```python
from build123d import *

# Parameters (mm, degrees)
BOSS_EXTRUDE1_DEPTH = 12
SKETCH3_R           = 1.184698277
CUT_EXTRUDE3_DEPTH  = 5
BOSS_EXTRUDE6_DEPTH = 12
CUT_EXTRUDE4_DEPTH  = 12
SKETCH10_R          = 1.184698277
CUT_EXTRUDE5_DEPTH  = 12
CUT_EXTRUDE7_DEPTH  = 19


with BuildPart() as part:
    # Sketch1 → Boss-Extrude1 (new body)
    with BuildSketch(Plane.XY):
        with BuildLine():
            Line((-4.775747962, -5), (-3.406624892, -5))
            ThreePointArc((-3.406624892, -5), (-6.090000101, 0), (-3.406624892, 5))
            Line((-3.406624892, 5), (3.226624689, 5))
            ThreePointArc((3.226624689, 5), (5.909999899, 0), (3.226624689, -5))
            Line((3.226624689, -5), (4.595747759, -5))
            ThreePointArc((4.595747759, -5), (-0.090000101, 6.852461821), (-4.775747962, -5))
        make_face()
        with BuildLine():
            Line((11.597073435, -5), (4.595747759, -5))
            ThreePointArc((4.595747759, -5), (3.939029098, -5.542847348), (3.220019991, -6))
            Line((3.220019991, -6), (11.597073435, -6))
            Line((11.597073435, -6), (11.597073435, -5))
        make_face()
        with BuildLine():
            Line((3.226624689, -5), (-3.406624892, -5))
            Line((-3.406624892, -5), (-4.775747962, -5))
            ThreePointArc((-4.775747962, -5), (-4.119029301, -5.542847348), (-3.400020194, -6))
            Line((-3.400020194, -6), (3.220019991, -6))
            ThreePointArc((3.220019991, -6), (3.939029098, -5.542847348), (4.595747759, -5))
            Line((4.595747759, -5), (3.226624689, -5))
        make_face()
        with BuildLine():
            ThreePointArc((-3.400020194, -6), (-4.119029301, -5.542847348), (-4.775747962, -5))
            Line((-4.775747962, -5), (-11.777073637, -5))
            Line((-11.777073637, -5), (-11.777073637, -6))
            Line((-11.777073637, -6), (-3.400020194, -6))
        make_face()
    extrude(amount=BOSS_EXTRUDE1_DEPTH)

    # Sketch3 → Cut-Extrude3 (cut)
    with BuildSketch(Plane(origin=(0, -5, 0), x_dir=(1, 0, 0), z_dir=(0, 1, 0))):
        with Locations((-9.627163284, -9.379788166)):
            Circle(SKETCH3_R)
        with Locations((9.447163082, -9.379788166)):
            Circle(SKETCH3_R)
        with Locations((9.447163082, -2.620211834)):
            Circle(SKETCH3_R)
        with Locations((-9.627163284, -2.620211834)):
            Circle(SKETCH3_R)
    extrude(amount=-CUT_EXTRUDE3_DEPTH, mode=Mode.SUBTRACT)

    # Sketch7 → Boss-Extrude6 (add)
    with BuildSketch(Plane.XY.offset(12)):
        with BuildLine():
            ThreePointArc((5.456145908, -5), (0, 7.400643767), (-5.456145908, -5))
            Line((-5.456145908, -5), (-4.775747962, -5))
            ThreePointArc((-4.775747962, -5), (-0.090000101, 6.852461821), (4.595747759, -5))
            Line((4.595747759, -5), (5.456145908, -5))
        make_face()
        with BuildLine():
            Line((-4.33238135, -6), (-11.777073637, -6))
            Line((-11.777073637, -6), (-11.777073637, -6.756480667))
            Line((-11.777073637, -6.756480667), (-3.019850519, -6.756480667))
            ThreePointArc((-3.019850519, -6.756480667), (-3.695523524, -6.411913447), (-4.33238135, -6))
        make_face()
        with BuildLine():
            Line((4.33238135, -6), (-4.33238135, -6))
            ThreePointArc((-4.33238135, -6), (-3.695523524, -6.411913447), (-3.019850519, -6.756480667))
            Line((-3.019850519, -6.756480667), (3.019850519, -6.756480667))
            ThreePointArc((3.019850519, -6.756480667), (3.695523524, -6.411913447), (4.33238135, -6))
        make_face()
        with BuildLine():
            Line((11.597073435, -6), (4.33238135, -6))
            ThreePointArc((4.33238135, -6), (3.695523524, -6.411913447), (3.019850519, -6.756480667))
            Line((3.019850519, -6.756480667), (11.597073435, -6.756480667))
            Line((11.597073435, -6.756480667), (11.597073435, -6))
        make_face()
    extrude(amount=-BOSS_EXTRUDE6_DEPTH)

    # Sketch9 → Cut-Extrude4 (cut)
    with BuildSketch(Plane.XY.offset(12)):
        with BuildLine():
            Line((-3.476794678, 5), (3.476794678, 5))
            ThreePointArc((3.476794678, 5), (6.090000101, 0), (3.476794678, -5))
            Line((3.476794678, -5), (-3.476794678, -5))
            ThreePointArc((-3.476794678, -5), (-6.090000101, 0), (-3.476794678, 5))
        make_face()
    extrude(amount=-CUT_EXTRUDE4_DEPTH, mode=Mode.SUBTRACT)

    # Sketch10 → Cut-Extrude5 (cut)
    with BuildSketch(Plane(origin=(0, -5, 0), x_dir=(1, 0, 0), z_dir=(0, 1, 0))):
        with Locations((-9.627163284, -2.620211834)):
            Circle(SKETCH10_R)
        with Locations((-9.627163284, -9.379788166)):
            Circle(SKETCH10_R)
        with Locations((9.447163082, -2.620211834)):
            Circle(SKETCH10_R)
        with Locations((9.447163082, -9.379788166)):
            Circle(SKETCH10_R)
    extrude(amount=-CUT_EXTRUDE5_DEPTH, mode=Mode.SUBTRACT)

    # Sketch11 → Cut-Extrude7 (cut)
    with BuildSketch(Plane.XY.offset(12)):
        with BuildLine():
            Line((-3.476794678, 5), (-3.871774203, 5))
            ThreePointArc((-3.871774203, 5), (-6.323814947, 0), (-3.871774203, -5))
            Line((-3.871774203, -5), (-3.476794678, -5))
            Line((-3.476794678, -5), (3.871774203, -5))
            ThreePointArc((3.871774203, -5), (6.323814947, 0), (3.871774203, 5))
            Line((3.871774203, 5), (-3.476794678, 5))
        make_face()
    extrude(amount=-CUT_EXTRUDE7_DEPTH, mode=Mode.SUBTRACT)


solid = part.part
```
Geometry: final body of the model. Coordinates: model frame, mm. A direction names the side the tool comes from. Round coordinates to 2 decimals unless told otherwise and drop trailing zeros. Write each loop counter-clockwise with the first axis right and the second up, starting at its lowest first coordinate (ties: lowest second). Pieces come first, ordered by that corner, then holes. Notation, with made-up numbers: M -10.75,39.5 L 29.25,39.5 A29 ccw 29.25,62.5 Z; hole C 59,-39 d3. An arc over 180 degrees is marked long. Answer in a Markdown table with one row per item. Add a question column.
(1) Draft query along X for faces 1 (the face through (-10.81, -5.87, 2.57)), 2 (the face through (0, -5, 6)), 3 (the face through (11.597, -6, 6)), 4 (the face through (-0.1, -5.4, 0)). Return one class per face: pulls with the +X half, pulls with the -X half, needs draft (parallel to the pull), parting line crosses it, or undercut.
(2) Cut plane B-B, the plane z = 7. Return the cut outline in (x, y), then the cut area to 3 significant figures.
(3) Reachability of faces 5 (the face through (-9, -5, 6)), 6 (the face through (9, -5, 6)), 7 (the face through (8.574, -5.866, 1.82)), 8 (the face through (-0.1, -5.4, 12)), 9 (the face through (0, 5, 6)) from +Z, -Z, +X, -X, +Y, -Y: full face, straight path, thin tool, end or side. Return the list, or none.
(4) Contact query for flat-ended pins moving along their axis: pin 1 (2 mm diameter, centred on x = 0, y = -2.5, fed in from -Z); pin 2 (2 mm diameter, centred on y = 0, z = 10, fed in from +X); pin 3 (1.9 mm diameter, centred on x = -9.5, z = 7.5, fed in from +Y); pin 4 (5 mm diameter, centred on x = 8, z = 6, fed in from +Y). Output: stop coordinate, or through.
(5) Cut plane C-C, the plane x = 0. Return the cut outline in (y, z).
(6) Ray query, L1, parallel to X at y = 0.25, z = 6.25; L2, parallel to Y at x = -5.75, z = 4.25; L3, parallel to Y at x = -8.75, z = 7.25. Return the intervals inside material, ascending.
(7) Cut plane A-A, the plane y = 0. Return the cut outline in (x, z), then the cut area to 3 significant figures.
(8) Cut plane D-D, the plane z = 9.75. Return the cut outline in (x, y), then the cut area to 3 significant figures.
Established:
| question | item | result |
|---|---|---|
| 1 | face 1 | undercut |
| 1 | face 2 | undercut |
| 1 | face 3 | pulls with the +X half |
| 1 | face 4 | needs draft |
| 2 | outline | M -11.78,-6.76 L 11.6,-6.76 L 11.6,-5 L 5.46,-5 A7.4 ccw long -5.46,-5 L -11.78,-5 Z; hole M -3.87,-5 L 3.87,-5 A6.32 ccw 3.87,5 L -3.87,5 A6.32 ccw Z |
| 2 | area | 83.3 mm² |
| 3 | face 5 | +Z, -Z, -X |
| 3 | face 6 | +Z, -Z, +X |
| 3 | face 7 | +Y, -Y |
| 3 | face 8 | +Z, +X, -X, +Y, -Y |
| 3 | face 9 | +Z, -Z |
| 4 | pin 1 | through |
| 4 | pin 2 | x = 7.4 |
| 4 | pin 3 | y = -5 |
| 4 | pin 4 | y = 4.95 |
| 5 | outline | M -6.76,0 L -5,0 L -5,12 L -6.76,12 Z; M 5,0 L 7.4,0 L 7.4,12 L 5,12 Z |
| 6 | L1 | -7.4 to -6.32, 6.32 to 7.4 |
| 6 | L2 | -6.76 to -5, -4.66 to -2.63, 2.63 to 4.66 |
| 6 | L3 | -6.76 to -5 |
| 7 | outline | M -7.4,0 L -6.32,0 L -6.32,12 L -7.4,12 Z; M 6.32,0 L 7.4,0 L 7.4,12 L 6.32,12 Z |
| 7 | area | 25.8 mm² |
| 8 | outline | M -11.78,-6.76 L -10.75,-6.76 L -10.75,-5 L -11.78,-5 Z; M -8.5,-6.76 L 8.32,-6.76 L 8.32,-5 L 5.46,-5 A7.4 ccw long -5.46,-5 L -8.5,-5 Z; M 10.57,-6.76 L 11.6,-6.76 L 11.6,-5 L 10.57,-5 Z; hole M -3.87,-5 L 3.87,-5 A6.32 ccw 3.87,5 L -3.87,5 A6.32 ccw Z |
| 8 | area | 75.4 mm² |
